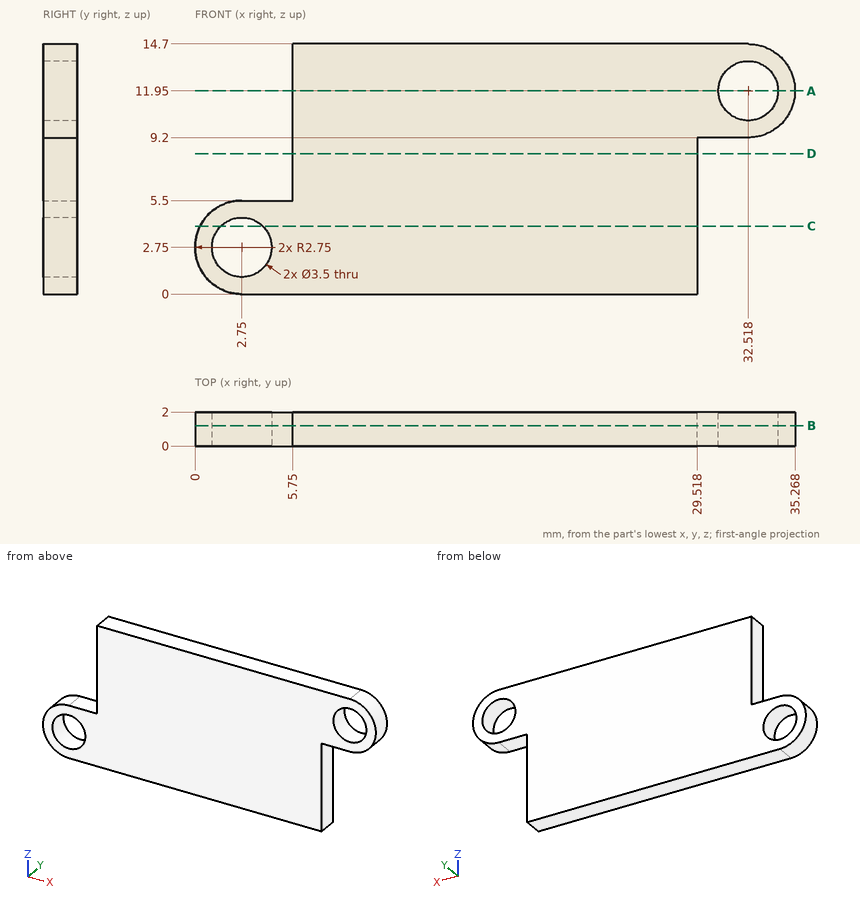
The figure shows three views and two pictorial views of one solid part (mm, origin at its lowest corner). Answer the questions. Coordinates: 2 decimals unless noted, no trailing zeros. Order: outer loops, then holes, each group sorted by start corner. A loop starts at its lowest first (then second) coordinate and runs counter-clockwise, first axis right, second up.
Q1. A cutting plane is placed at B-B, the plane y = 1.2. Write down the section's boundary in (x, z), and give its area (3 significant figures).
Q2. Consider line 1 (Z direction, x = 2.75, y = 1.55); line 2 (Z direction, x = 32, y = 1); line 3 (X direction, y = 1.85, z = 3.5) (1 decimal). Determine where each line is inside the solid, lowest interval first.
Q3. A cutting plane is placed at A-A, the plane z = 11.95. Write down the section's boundary in (x, y).
Q4. A cutting plane is placed at C-C, the plane z = 4. Write down the section's boundary in (x, y) (1 decimal).
Q5. A cutting plane is placed at D-D, the plane z = 8.25. Write down the section's boundary in (x, y).
Q6. Given P1, Ø3, axis at x = 2.75, z = 2.75, coming from the -Y side; P2, Ø1, axis at x = 31, y = 1, coming from the -Z side; P3, Ø1, axis at y = 1, z = 4.5, coming from the +X side, each flat-ended and moving along its own axis, determine where each tip first touches the part or whether it passes through.
Answers follow:
1. outline: (2.75, 0) - (29.52, 0) - (29.52, 9.2) - (32.52, 9.2) arc R2.75 ccw to (32.52, 14.7) - (5.75, 14.7) - (5.75, 5.5) - (2.75, 5.5) arc R2.75 ccw to start; hole circle Ø3.5 at (2.75, 2.75); hole circle Ø3.5 at (32.52, 11.95)
1. area: 387 mm2
2. line 1: z = 0 to 1, 4.5 to 5.5
2. line 2: z = 9.2 to 10.28, 13.62 to 14.7
2. line 3: x = 0.1 to 1.2, 4.3 to 29.5
3. outline: (5.75, 0) - (30.77, 0) - (30.77, 2) - (5.75, 2) - close; (34.27, 0) - (35.27, 0) - (35.27, 2) - (34.27, 2) - close
4. outline: (0.3, 0) - (1.5, 0) - (1.5, 2) - (0.3, 2) - close; (4, 0) - (29.5, 0) - (29.5, 2) - (4, 2) - close
5. outline: (5.75, 0) - (29.52, 0) - (29.52, 2) - (5.75, 2) - close
6. P1: passes through
6. P2: stops at z = 9.2
6. P3: stops at x = 29.52
